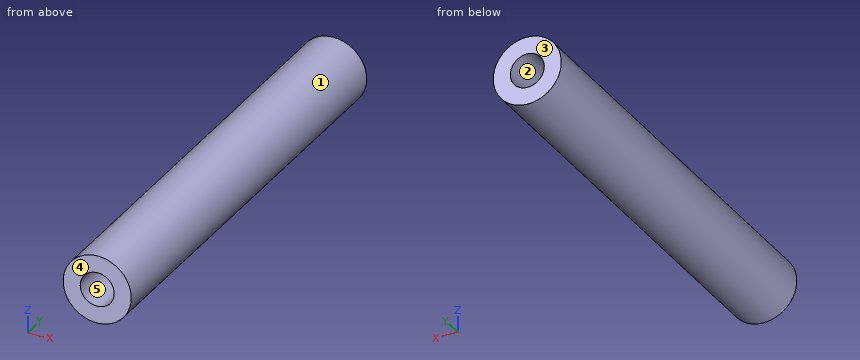
Autodesk Fusion 360 part; units mm, degrees
sketch "Boceto1" plane through (0, 0, 0) normal (0, 1, 0) x (1, 0, 0)
  circle A0 centre (0, 0) radius 3
  dimension "d1" = 6
extrude "Extruir1" add sketch "Boceto1" along normal blind 40
sketch "Boceto2" plane through (0, 40, 0) normal (0, 1, 0) x (-1, 0, 0)
  circle A0 centre (0, 0) radius 3
  circle A1 centre (0, 0) radius 1.525
  dimension "d4" = 3.05
sketch "Boceto3" plane through (0, 0, 0) normal (0, -1, 0) x (1, 0, 0)
  circle A0 centre (0, 0) radius 3
  circle A1 centre (0, 0) radius 1.525
  dimension "d5" = 3.05
hole "Agujero1" at (0, 40, 0) direction (0, -1, 0) diameter 3 depth 10 tip angle 118
hole "Agujero2" at (0, 0, 0) direction (0, 1, 0) diameter 3 depth 10 tip angle 118
Source: CAD feature listing. Evaluate the final solid. Frame: model axes, mm. Face numbers are marked on the shaded views. A direction names the side the tool comes from. Give positions to 0.01 mm unless a question says otherwise; leave off trailing zeros. Loops run counter-clockwise (first coordinate to the right, second up) from the corner with the lowest first, then second, coordinate; pieces in that order, holes last. Notation, with made-up numbers: M -6.75,-33.5 L 11.25,-33.5 A12 ccw 11.25,-13.5 Z; hole C -13.5,12.5 d8. An arc over 180 degrees is marked long. Put each result on its own line as item: value.
Q1. Section C-C (x = -2.3). Return the cut outline in (y, z), and give its area (3 significant figures).
Response values:
outline: M 0,-1.93 L 40,-1.93 L 40,1.93 L 0,1.93 Z
area: 154 mm²
Q2. Section A-A (y = 33.5). Return the cut outline in (x, z).
Response values:
outline: C 0,0 d6; hole C 0,0 d3
Q3. Section B-B (y = 14). Return the cut outline in (x, z).
Response values:
outline: C 0,0 d6
Q4. Reachability of the marked faces 4 and 5 from +Z, -Z, +X, -X, +Y, -Y: full face, straight path, thin tool, end or side. Return the list, or none.
Response values:
face 4: +Z, -Z, +X, -X, -Y
face 5: -Y
Q5. Line query: probe 1 along X at (y, z) = (2, 0); probe 2 along X at (y, z) = (8.5, 0.5). Output: solid intervals per line, ascending. Write a range as [from, to].
Response values:
probe 1: x = [-3, -1.5], [1.5, 3]
probe 2: x = [-2.96, -1.41], [1.41, 2.96]
Q6. Pin query (flat end, axial travel): P1, Ø1.5, axis at y = 15, z = -2, coming from the -X side; P2, Ø1.5, axis at x = 0.5, z = 0.5, coming from the -Y side; P3, Ø2.5, axis at x = 0, z = 0, coming from the -Y side. Return the tip coordinate at first contact, or that it passes through.
Response values:
P1: stops at x = -2.73
P2: stops at y = 10.03
P3: stops at y = 10.15
Q7. Section D-D (z = 2.2). Return the cut outline in (x, y), and give its area (3 significant figures).
Response values:
outline: M -2.04,0 L 2.04,0 L 2.04,40 L -2.04,40 Z
area: 163 mm²
Q8. Mould query, pull axis X, two halves, no side actions, for the marked faces 1, 2 and 3. Classes: released by +X, released by -X, zero draft, split by the parting line, or undercut.
Response values:
face 1: split by the parting line
face 2: undercut
face 3: zero draft
